Can you work these out from the model? Positions are in its coordinate system, mm. A direction names the side the tool comes from. Give positions to 0.01 mm unless a question says otherwise; leave off trailing zeros. Answer as a JSON object with one key per item and string values.
```python
from build123d import *

# Parameters (mm, degrees)
F1_DEPTH = 76.2
F2_R     = 38.1
F3_R     = 1.27
F4_R     = 13.3186295464
F5_DEPTH = 50.8010001


with BuildPart() as f1:
    # F0 (on Top) → F1 (new body)
    with BuildSketch(Plane.XY):
        with BuildLine():
            Line((50.8, -38.1), (50.8, 38.1))
            add(Edge.make_bspline(
                [(-50.8, 0), (-42.9578186496, 7.6088566123), (-27.7925786216, 22.3228909539), (-0.3325914479, 21.3832091321), (34.1809209144, 21.8501210604), (45.6546344586, 33.0689548857), (50.8, 38.1)],
                knots=[0, 0, 0, 0, 0.2616576069, 0.5059943202, 0.7784647329, 1, 1, 1, 1], degree=3))
            Line((-50.8, 0), (-50.8, -38.1))
            Line((-50.8, -38.1), (50.8, -38.1))
        make_face()
    extrude(amount=F1_DEPTH)

    # F2
    f2_edges = [f1.edges().sort_by_distance(p)[0] for p in [
        (50.8, -38.1, 38.1),
        (-50.8, 0, 38.1),
    ]]
    fillet(f2_edges, radius=F2_R)

    # F3
    f3_edges = [f1.edges().sort_by_distance(p)[0] for p in [
        (9.791993, 21.686914, 76.2),
        (-19.05, -38.1, 76.2),
        (39.640768, -26.940768, 76.2),
        (-19.05, -38.1, 0),
        (9.791993, 21.686914, 0),
    ]]
    fillet(f3_edges, radius=F3_R)

    # F4 (on Right) → F5 (cut, through all)
    with BuildSketch(Plane.YZ):
        with Locations((0, 39.7054702044)):
            Circle(F4_R)
    extrude(amount=-F5_DEPTH, mode=Mode.SUBTRACT)


solid = f1.part
```
1. If we mould it in two halves opening along Y, with no side actions, what happens to faces 1 (the face through (39.94, -26.64, 38.62)), 2 (the face through (-50.8, -27, 38)), 3 (the face through (0, 0, 40))? For each: +Y half, -Y half, draft (parallel to the pull), parting line (faces both ways), or undercut.
Worked answers:
{"face 1": "-Y half", "face 2": "draft", "face 3": "undercut"}
2. Will these pins go through, and if not, where does the flat tip stop? pin 1 Ø10 at (x, z) = (-26, 39.5) entering from +Y; pin 2 Ø3 at (x, z) = (28, 30) entering from +Y; pin 3 Ø4 at (x, z) = (28, 9.5) entering from +Y.
Worked answers:
{"pin 1": "y = 20.45", "pin 2": "y = 24.06", "pin 3": "y = 24.2"}
3. Please list where these lines run through material, in increasing order: L1, parallel to Z at x = -31, y = 0; L2, parallel to Y at x = 32.5, z = 57.5; L3, parallel to X at y = 14.5, z = 47.
Worked answers:
{"L1": "0 to 26.39, 53.02 to 76.2", "L2": "-32.55 to 25.01", "L3": "-34.19 to 50.8"}
4. For faces 4 (the face through (-24.959, -13.306, 40.291)), 5 (the face through (-19, -38.1, 38)), which set-ups out of +Z, -Z, +X, -X, +Y, -Y let a thin tool reach every point of the face, with its end or its side?
Worked answers:
{"face 4": "-X", "face 5": "+Z, -Z, +X, -X, -Y"}
